```python
from build123d import *

# Parameters (mm, degrees)
SKETCH1_W           = 76.2
SKETCH1_H           = 25.4
SKETCH1_W_2         = 70.104
SKETCH1_H_2         = 19.304
BOSS_EXTRUDE1_DEPTH = 305.4
CUT_EXTRUDE1_START  = -12.7
SKETCH3_W           = 76.2
SKETCH3_H           = 25.4
CUT_EXTRUDE1_DEPTH  = 25.4
CUT_EXTRUDE2_START  = -12.7
SKETCH4_W           = 76.2
SKETCH4_H           = 25.4
CUT_EXTRUDE2_DEPTH  = 25.4


with BuildPart() as part:
    # Sketch1 → Boss-Extrude1 (new body)
    with BuildSketch(Plane(origin=(0, 0, 0), x_dir=(1, 0, 0), z_dir=(0, 1, 0))):
        Rectangle(SKETCH1_W, SKETCH1_H)
        Rectangle(SKETCH1_W_2, SKETCH1_H_2, mode=Mode.SUBTRACT)
    extrude(amount=BOSS_EXTRUDE1_DEPTH)

    # Sketch3 → Cut-Extrude1 (cut)
    with BuildSketch(Plane.XY.offset(CUT_EXTRUDE1_START)):
        Rectangle(SKETCH3_W, SKETCH3_H)
    extrude(amount=CUT_EXTRUDE1_DEPTH, mode=Mode.SUBTRACT)

    # Sketch4 → Cut-Extrude2 (cut)
    with BuildSketch(Plane(origin=(0, 305.4, 0), x_dir=(1, 0, 0), z_dir=(0, 0, 1)).offset(CUT_EXTRUDE2_START)):
        Rectangle(SKETCH4_W, SKETCH4_H)
    extrude(amount=CUT_EXTRUDE2_DEPTH, mode=Mode.SUBTRACT)


solid = part.part
```
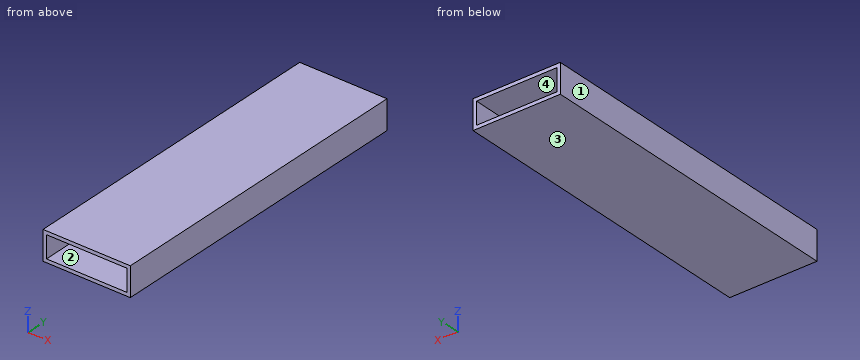
Build history of the part. All positions in model axes, mm. Face numbers are marked on the shaded views. Coordinates: 2 decimals unless noted, no trailing zeros. Order: outer loops, then holes, each group sorted by start corner. A loop starts at its lowest first (then second) coordinate and runs counter-clockwise, first axis right, second up.
Item 1: Saw through at B-B on x = -22.5. List the corners of the cut face in (y, z), then the cut area to 3 significant figures.
Filled in:
outline: (12.7, -12.7) - (292.7, -12.7) - (292.7, -9.65) - (12.7, -9.65) - close; (12.7, 9.65) - (292.7, 9.65) - (292.7, 12.7) - (12.7, 12.7) - close
area: 1,710 mm2
Item 2: Saw through at A-A on y = 90. List the corners of the cut face in (x, z), then the cut area to 3 significant figures.
Filled in:
outline: (-38.1, -12.7) - (38.1, -12.7) - (38.1, 12.7) - (-38.1, 12.7) - close; hole (-35.05, -9.65) - (35.05, -9.65) - (35.05, 9.65) - (-35.05, 9.65) - close
area: 582 mm2
Item 3: Mould opens along X. For the marked faces 1, 2, 3 and 4 say: released by +X, released by -X, zero draft, split by the parting line, or undercut.
Filled in:
face 1: released by -X
face 2: undercut
face 3: zero draft
face 4: undercut
Item 4: Drill centre lines: L1, parallel to Z at x = 16.5, y = 96; L2, parallel to X at y = 217, z = 3. Where is each one in solid material? Low to high.
Filled in:
L1: z = -12.7 to -9.65, 9.65 to 12.7
L2: x = -38.1 to -35.05, 35.05 to 38.1
Item 5: Saw through at C-C on z = 3.25. List the corners of the cut face in (x, y).
Filled in:
outline: (-38.1, 12.7) - (-35.05, 12.7) - (-35.05, 292.7) - (-38.1, 292.7) - close; (35.05, 12.7) - (38.1, 12.7) - (38.1, 292.7) - (35.05, 292.7) - close
Item 6: Drop a flat-ended pin along its axis: pin 1 Ø10 at (x, z) = (-13, 1) entering from -Y. Give the stop position or say it passes through.
Filled in:
pin 1: passes through
